Print and shaded views of the part. All mm, measured from the part's lowest x, y and z. Coordinates: 2 decimals unless noted, no trailing zeros. Order: outer loops, then holes, each group sorted by start corner. A loop starts at its lowest first (then second) coordinate and runs counter-clockwise, first axis right, second up.
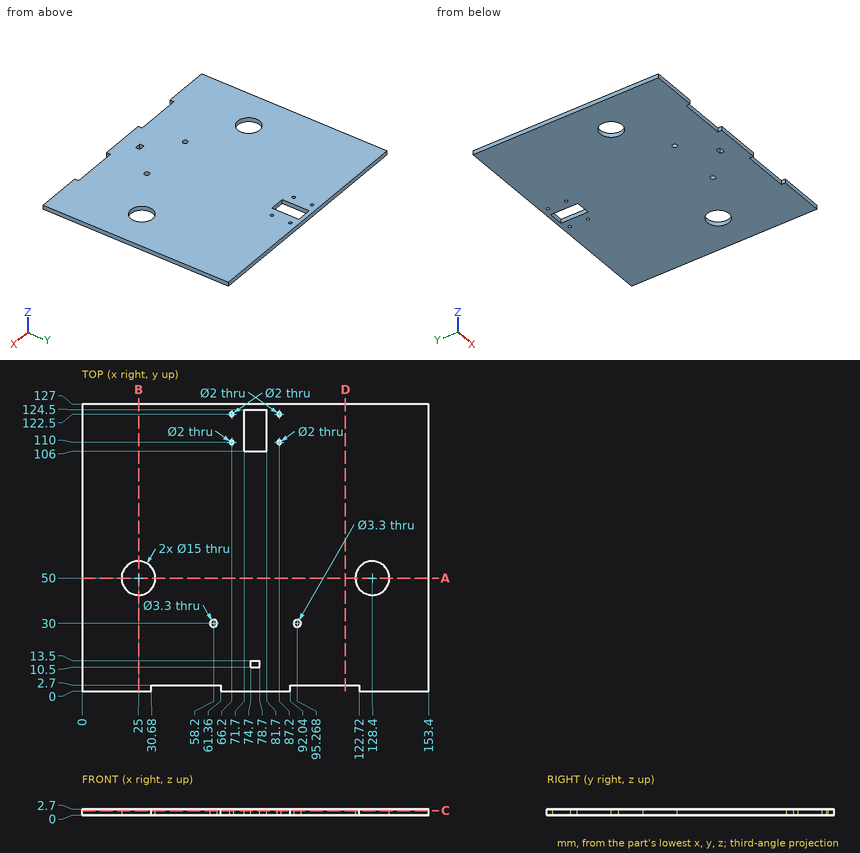
Q1. Cut at C-C, the plane z = 2.1. Count the separate pieces of the cut face and the enclosed holes in it, plus the area to 3 significant figures.
Established:
separate pieces: 1
enclosed holes: 10
area: 18,700 mm2
Q2. Drop flat-ended pins along their axis: P1, Ø12, axis at x = 25, y = 50, coming from the -Z side; P2, Ø1, axis at x = 49.5, z = 1.5, coming from the -Y side. Give the stop position or say it passes through.
Established:
P1: passes through
P2: stops at y = 2.7
Q3. Probe line 1 (X direction, y = 110, z = 1.35); line 2 (Y direction, x = 66.2, z = 1.4); line 3 (Y direction, x = 74, z = 1.45). List the from-to ranges inside material, lowest first.
Established:
line 1: x = 0 to 65.2, 67.2 to 71.7, 81.7 to 86.2, 88.2 to 153.4
line 2: y = 0 to 109, 111 to 121.5, 123.5 to 127
line 3: y = 0 to 106, 124.5 to 127
Q4. Cut at A-A, the plane y = 50. List the corners of the cut face in (x, z).
Established:
outline: (0, 0) - (17.5, 0) - (17.5, 2.7) - (0, 2.7) - close; (32.5, 0) - (120.9, 0) - (120.9, 2.7) - (32.5, 2.7) - close; (135.9, 0) - (153.4, 0) - (153.4, 2.7) - (135.9, 2.7) - close
Q5. Cut at D-D, the plane x = 116.5. List the corners of the cut face in (y, z).
Established:
outline: (2.7, 0) - (127, 0) - (127, 2.7) - (2.7, 2.7) - close
Q6. Cut at B-B, the plane x = 25. List the corners of the cut face in (y, z).
Established:
outline: (0, 0) - (42.5, 0) - (42.5, 2.7) - (0, 2.7) - close; (57.5, 0) - (127, 0) - (127, 2.7) - (57.5, 2.7) - close
